The listing builds one solid part. Answer for the finished solid, in the listing's coordinates (mm). Face numbers are marked on the shaded views. A direction names the side the tool comes from. Round coordinates to 2 decimals unless told otherwise and drop trailing zeros. Write each loop counter-clockwise with the first axis right and the second up, starting at its lowest first coordinate (ties: lowest second). Pieces come first, ordered by that corner, then holes.
from build123d import *

# Parameters (mm, degrees)
F1_DEPTH = 3.81
F2_W     = 6.35
F2_H     = 4.7692152426
F2_H_2   = 4.7557847574
F2_H_3   = 9.525
F2_W_2   = 4.0261267766
F3_DEPTH = 25.4
F4_R     = 1.7598288085
F4_R_2   = 1.7653
F5_DEPTH = 25.4
F7_DEPTH = 25.4


with BuildPart() as f1:
    # F0 (on Top) → F1 (new body)
    with BuildSketch(Plane.XY):
        with BuildLine():
            Line((-3.175, -15.875), (3.175, -15.875))
            ThreePointArc((3.175, -15.875), (7.6651280605, -14.0151280605), (9.525, -9.525))
            Line((9.525, -9.525), (9.525, 9.525))
            ThreePointArc((9.525, 9.525), (7.6651280605, 14.0151280605), (3.175, 15.875))
            Line((3.175, 15.875), (-3.175, 15.875))
            ThreePointArc((-3.175, 15.875), (-7.6651280605, 14.0151280605), (-9.525, 9.525))
            Line((-9.525, 9.525), (-9.525, -9.525))
            ThreePointArc((-9.525, -9.525), (-7.6651280605, -14.0151280605), (-3.175, -15.875))
        make_face()
    extrude(amount=F1_DEPTH)

    # F2 (on face) → F3 (cut)
    with BuildSketch(Plane.XY.offset(3.81)):
        with Locations((0, 7.1403923787)):
            Rectangle(F2_W, F2_H)
        with Locations((0, 2.3778923787)):
            Rectangle(F2_W, F2_H_2)
        with Locations((0, -4.7625)):
            Rectangle(F2_W, F2_H_3)
        with Locations((-5.1880633883, 2.3778923787)):
            Rectangle(F2_W_2, F2_H_2)
        with Locations((5.1880633883, 2.3778923787)):
            Rectangle(F2_W_2, F2_H_2)
    extrude(amount=-F3_DEPTH, mode=Mode.SUBTRACT)

    # F4 (on face) → F5 (cut)
    with BuildSketch(Plane.XY.offset(3.81)):
        with Locations((0, 13.2097881287)):
            Circle(F4_R)
        with Locations((4.7985878773, 12.0691694319)):
            Circle(F4_R_2)
        with Locations((-4.7985878773, 12.0691694319)):
            Circle(F4_R_2)
        with Locations((-4.7985878773, -12.0691694319)):
            Circle(F4_R_2)
        with Locations((0, -13.2097881287)):
            Circle(F4_R)
        with Locations((4.7985878773, -12.0691694319)):
            Circle(F4_R_2)
    extrude(amount=-F5_DEPTH, mode=Mode.SUBTRACT)

    # F6 (on face) → F7 (cut)
    with BuildSketch(Plane.XY.offset(3.81)):
        Polygon((6.372133691, -5.9245415708), (8.7422396946, -4.5306024468), (8.7201060036, -1.7810608759), (6.327866309, -0.4254584292), (3.9577603054, -1.8193975532), (3.9798939964, -4.5689391241), align=None)
    extrude(amount=-F7_DEPTH, mode=Mode.SUBTRACT)


solid = f1.part
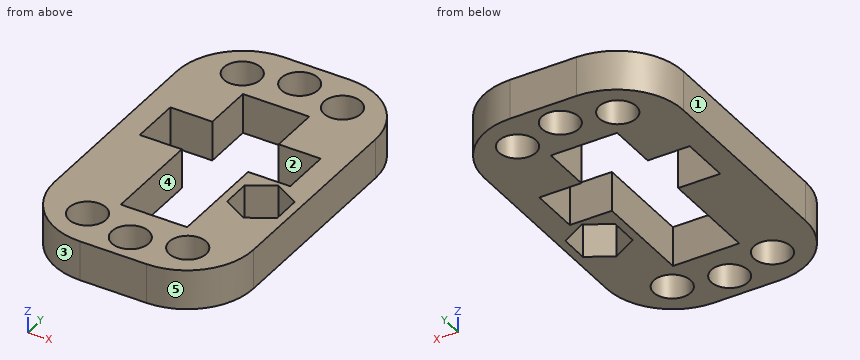
1. Section B-B on x = 0 is taken. Determine the outline of the cut face in (y, z) (3 decimals), plus the area to 3 significant figures.
Geometry says:
outline: (-15.875, 0) - (-14.97, 0) - (-14.97, 3.81) - (-15.875, 3.81) - close; (-11.45, 0) - (-9.525, 0) - (-9.525, 3.81) - (-11.45, 3.81) - close; (9.525, 0) - (11.45, 0) - (11.45, 3.81) - (9.525, 3.81) - close; (14.97, 0) - (15.875, 0) - (15.875, 3.81) - (14.97, 3.81) - close
area: 21.6 mm2
2. For a pull along Y with two mould halves and no side action, classify the marked faces 1, 2 and 3 as released by +Y, released by -Y, zero draft, split by the parting line, or undercut.
Geometry says:
face 1: zero draft
face 2: undercut
face 3: released by -Y
3. A tool of negligible diameter and unlimited length cuts with its end or side. For the marked faces 4 and 5, from which of +Z, -Z, +X, -X, +Y, -Y can it reach the whole face along a straight path? Write none if from no direction.
Geometry says:
face 4: +Z, -Z
face 5: +Z, -Z, +X, -Y
4. Straight lines are drawn through the part: line 1 along Y through (x, z) = (0, 0.35) (3 decimals); line 2 along X through (y, z) = (-8, 3.1) (3 decimals); line 3 along Y through (x, z) = (1.5, 1.75) (3 decimals). For each, find the intervals that lie inside material, in ascending order.
Geometry says:
line 1: y = -15.875 to -14.97, -11.45 to -9.525, 9.525 to 11.45, 14.97 to 15.875
line 2: x = -9.525 to -3.175, 3.175 to 9.525
line 3: y = -15.875 to -14.13, -12.289 to -9.525, 9.525 to 12.289, 14.13 to 15.875
5. Given pin 1 (1.9 mm diameter, centred on x = -5, z = 2, fed in from -Y); pin 2 (4 mm diameter, centred on x = -5, y = 7, fed in from -Z), each flat-ended and moving along its own axis, determine where each tip first touches the part or whether it passes through.
Geometry says:
pin 1: stops at y = -15.81
pin 2: stops at z = 0
6. Section C-C on y = -12.5 is taken. Determine the outline of the cut face in (x, z), plus the area to 3 significant figures.
Geometry says:
outline: (-8.78, 0) - (-6.51, 0) - (-6.51, 3.81) - (-8.78, 3.81) - close; (-3.09, 0) - (-1.61, 0) - (-1.61, 3.81) - (-3.09, 3.81) - close; (1.61, 0) - (3.09, 0) - (3.09, 3.81) - (1.61, 3.81) - close; (6.51, 0) - (8.78, 0) - (8.78, 3.81) - (6.51, 3.81) - close
area: 28.6 mm2
7. Section A-A on y = -7 is taken. Determine the outline of the cut face in (x, z) (3 decimals).
Geometry says:
outline: (-9.525, 0) - (-3.175, 0) - (-3.175, 3.81) - (-9.525, 3.81) - close; (3.175, 0) - (9.525, 0) - (9.525, 3.81) - (3.175, 3.81) - close
8. Section D-D on z = 1.4 is taken. Give the number of separate pieces and of enclosed holes in the cut face, plus the area to 3 significant figures.
Geometry says:
separate pieces: 1
enclosed holes: 8
area: 333 mm2
